from build123d import *

# Parameters (mm, degrees)
F0_W     = 6
F0_H     = 6
F1_DEPTH = 6
F2_W     = 7
F2_H     = 7
F3_DEPTH = 1
F4_W     = 7
F4_H     = 7
F5_DEPTH = 1
F6_W     = 6
F6_H     = 0.5
F7_DEPTH = 8.001


with BuildPart() as f1:
    # F0 (on Top) → F1 (new body)
    with BuildSketch(Plane.XY):
        Rectangle(F0_W, F0_H)
    extrude(amount=F1_DEPTH)

    # F2 (on face) → F3 (join)
    with BuildSketch(Plane.XY.offset(6)):
        Rectangle(F2_W, F2_H)
    extrude(amount=F3_DEPTH)

    # F4 (on face) → F5 (join)
    with BuildSketch(Plane(origin=(0, 0, 0), x_dir=(1, 0, 0), z_dir=(0, 0, -1))):
        Rectangle(F4_W, F4_H)
    extrude(amount=F5_DEPTH)

    # F6 (on face) → F7 (cut, through all)
    with BuildSketch(Plane.XY.offset(7)):
        with Locations((0, 3.25)):
            Rectangle(F6_W, F6_H)
        with Locations((0, -3.25)):
            Rectangle(F6_W, F6_H)
    extrude(amount=-F7_DEPTH, mode=Mode.SUBTRACT)


solid = f1.part
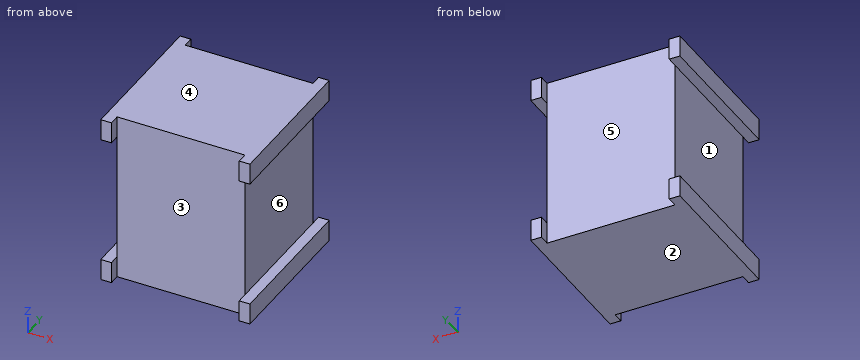
Part model, mm, in its own coordinate system. Face numbers are marked on the shaded views. A direction names the side the tool comes from. Give positions to 0.01 mm unless a question says otherwise; leave off trailing zeros. Loops run counter-clockwise (first coordinate to the right, second up) from the corner with the lowest first, then second, coordinate; pieces in that order, holes last. Notation, with made-up numbers: M 62.5,27 L 100.5,27 A16 cw 100.5,46 Z; hole C 0,-40 d4. An arc over 180 degrees is marked long. Put each result on its own line as item: value. Start each with the question number.
1) Flat gauge pins, fed straight in: pin 1 (3 mm diameter, centred on y = 0, z = 2, fed in from -X); pin 2 (1.5 mm diameter, centred on x = 1.5, z = 5.5, fed in from +Y); pin 3 (3 mm diameter, centred on y = -1, z = 3.5, fed in from +X). Where does each tip first touch, or does it go through?
2) Saw through at B-B (y = 1). List the corners of the cut face in (x, z), then the cut area to 3 significant figures.
3) Probe probe 1 along X at (y, z) = (1.25, 1.25). List the from-to ranges inside material, lowest first.
4) Pull direction Z, two halves, no side cores. Call the marked faces 4, 5 and 6: +Z half, -Z half, draft (parallel to the pull), parting line (faces both ways), or undercut.
5) Saw through at D-D (z = 5.75). List the corners of the cut face in (x, y), then the cut area to 3 significant figures.
6) Saw through at A-A (z = 6.75). List the corners of the cut face in (x, y), then the cut area to 3 significant figures.
7) Saw through at C-C (x = 1.25). List the corners of the cut face in (y, z), then the cut area to 3 significant figures.
8) 3-axis set-ups, long thin cutter, end or side, ignore diameter. For the marked faces 1, 2 and 3: which of +Z, -Z, +X, -X, +Y, -Y reach the whole face in a straight line?
Numbers:
1. pin 1: x = -3
1. pin 2: y = 3
1. pin 3: x = 3
2. outline: M -3.5,-1 L 3.5,-1 L 3.5,0 L 3,0 L 3,6 L 3.5,6 L 3.5,7 L -3.5,7 L -3.5,6 L -3,6 L -3,0 L -3.5,0 Z
2. area: 50.0 mm^2
3. probe 1: -3 to 3
4. face 4: +Z half
4. face 5: draft
4. face 6: undercut
5. outline: M -3,-3 L 3,-3 L 3,3 L -3,3 Z
5. area: 36.0 mm^2
6. outline: M -3.5,-3.5 L -3,-3.5 L -3,-3 L 3,-3 L 3,-3.5 L 3.5,-3.5 L 3.5,3.5 L 3,3.5 L 3,3 L -3,3 L -3,3.5 L -3.5,3.5 Z
6. area: 43.0 mm^2
7. outline: M -3,-1 L 3,-1 L 3,7 L -3,7 Z
7. area: 48.0 mm^2
8. face 1: -X, +Y, -Y
8. face 2: -Z, +X, -X, +Y, -Y
8. face 3: +Z, -Z, -Y
